Autodesk Inventor part; units mm, degrees
ref_plane "YZ Plane" through (0, 0, 0) normal (1, 0, 0) x (0, 1, 0)
ref_plane "XZ Plane" through (0, 0, 0) normal (0, 1, 0) x (-1, 0, 0)
ref_plane "XY Plane" through (0, 0, 0) normal (0, 0, 1) x (1, 0, 0)
sketch "スケッチ1" plane through (0, 0, 0) normal (0, 0, 1) x (1, 0, 0)
  circle A0 centre (0, 0) radius 2.55
  dimension "d0" = 5.1
extrude "押し出し1" add sketch "スケッチ1" along normal blind 1.2
sketch "スケッチ2" plane through (0, 0, 0) normal (0, 0, -1) x (-1, 0, 0)
  circle A0 centre (0, 0) radius 2.55
  circle A1 centre (0, 0) radius 1.5
  dimension "d3" = 3
extrude "押し出し2" add sketch "スケッチ2" along normal blind 10 contours A1
thread "ねじ1"
sketch "スケッチ3" plane through (0, 0, 1.2) normal (0, 0, 1) x (1, 0, 0)
  circle A0 centre (0, 0) radius 2.55
  line L0 (0, 1.1547) -> (1, 0.5774)
  line L1 (1, 0.5774) -> (1, -0.5774)
  line L2 (1, -0.5774) -> (0, -1.1547)
  line L3 (0, -1.1547) -> (-1, -0.5774)
  line L4 (-1, -0.5774) -> (-1, 0.5774)
  line L5 (-1, 0.5774) -> (0, 1.1547)
  dimension "d8" = 2
extrude "押し出し3" cut sketch "スケッチ3" against normal blind 1 contours L0 L1 L2 L3 L4 L5
fillet "フィレット1" radius 0.2 2 edges at (-2.55, 0, 1.2) (-2.55, 0, 0)
chamfer "面取り1" distance 0.2 angle 45 1 edges at (1.5, 0, -10)
properties part number "六角穴付低頭平 M3 x 10" material "鋼"
Build history of the part. All positions in model axes, mm. A direction names the side the tool comes from. Give positions to 0.01 mm unless a question says otherwise; leave off trailing zeros. Order: outer loops, then holes, each group sorted by start corner. A loop starts at its lowest first (then second) coordinate and runs counter-clockwise, first axis right, second up. Notation, with made-up numbers: M 76,34 L 96,34 A26 ccw 96,68 Z; hole C 42,-34 d11. An arc over 180 degrees is marked long. Return JSON: item names as keys, results as strings.
Q1. Flat gauge pins, fed straight in: pin 1 (2 mm diameter, centred on y = 1.5, z = -4, fed in from -X); pin 2 (2 mm diameter, centred on y = -0.5, z = -3, fed in from +X); pin 3 (1.6 mm diameter, centred on x = 0, y = 0, fed in from +Z). Where does each tip first touch, or does it go through?
Answer list:
{"pin 1": "stops at x = -1.41", "pin 2": "stops at x = 1.5", "pin 3": "stops at z = 0.2"}
Q2. 3-axis set-ups, long thin cutter, end or side, ignore diameter. For faces 4 (the face through (-0.49, -0.87, 0.71)), 5 (the face through (-1, -1, 1.2)): which of +Z, -Z, +X, -X, +Y, -Y reach the whole face in a straight line?
Answer list:
{"face 4": "+Z", "face 5": "+Z, +X, -X, +Y, -Y"}
Q3. Two-plate mould, pull along X, no slides. Class faces 1 (the face through (0, -2, 0)), 2 (the face through (1.5, -0.07, -4.83)), 3 (the face through (0.51, -0.86, 0.71)): pulls with the +X half, pulls with the -X half, needs draft (parallel to the pull), parting line crosses it, or undercut.
Answer list:
{"face 1": "needs draft", "face 2": "parting line crosses it", "face 3": "undercut"}
Q4. Band-saw the part on B-B (z = -3.25). Give the cut face in (x, y), then the cut area to 3 significant figures.
Answer list:
{"outline": "C 0,0 d3", "area": "7.07 mm^2"}
Q5. Band-saw the part on A-A (y = 0). Give the cut face in (x, z), then the cut area to 3 significant figures.
Answer list:
{"outline": "M -2.55,0.2 A0.2 ccw -2.35,0 L -1.5,0 L -1.5,-9.8 L -1.3,-10 L 1.3,-10 L 1.5,-9.8 L 1.5,0 L 2.35,0 A0.2 ccw 2.55,0.2 L 2.55,1 A0.2 ccw 2.35,1.2 L 1,1.2 L 1,0.2 L -1,0.2 L -1,1.2 L -2.35,1.2 A0.2 ccw -2.55,1 Z", "area": "34.0 mm^2"}
Q6. Wall check: probe 1 along Z at (x, y) = (0.75, 0); probe 2 along Z at (x, y) = (0.05, -1.85); probe 3 along Y at (x, z) = (0.3, 0.5). Give the ranges that are in metal, low to high. Write a range as from..to.
Answer list:
{"probe 1": "z = -10..0.2", "probe 2": "z = 0..1.2", "probe 3": "y = -2.53..-0.98, 0.98..2.53"}
